```python
from build123d import *

# Parameters (mm, degrees)
F0_W     = 60.96
F0_H     = 31.75
F1_DEPTH = 3.175
F2_R     = 5.08


# Not quite as in the source:
# - a length typed as a fraction of an inch, garbled in the dataset ("3 / 203.2 mm" for 3/8 in), is restored


with BuildPart() as f1:
    # F0 (on Top) → F1 (new body)
    with BuildSketch(Plane.XY):
        Rectangle(F0_W, F0_H)
        with BuildLine():
            Line((-8.128, -4.9660085582), (-8.128, 4.9660085582))
            ThreePointArc((-8.128, 4.9660085582), (0, 9.525), (8.128, 4.9660085582))
            Line((8.128, 4.9660085582), (8.128, -4.9660085582))
            ThreePointArc((8.128, -4.9660085582), (0, -9.525), (-8.128, -4.9660085582))
        make_face(mode=Mode.SUBTRACT)
    extrude(amount=F1_DEPTH)

    # F2
    f2_edges = [f1.edges().sort_by_distance(p)[0] for p in [
        (-30.48, 15.875, 1.5875),
        (30.48, 15.875, 1.5875),
        (-30.48, -15.875, 1.5875),
        (30.48, -15.875, 1.5875),
    ]]
    fillet(f2_edges, radius=F2_R)


solid = f1.part
```
Check sheet for the modelled part. Datum: model origin and axes. Units: mm. A direction names the side the tool comes from. Coordinates: 2 decimals unless noted, no trailing zeros. Order: outer loops, then holes, each group sorted by start corner. A loop starts at its lowest first (then second) coordinate and runs counter-clockwise, first axis right, second up. Notation, with made-up numbers: M -29,5 L 4,5 A25 ccw 4,43 Z; hole C 48,1.25 d8. An arc over 180 degrees is marked long. One line per question, with ' | ' between items. Start each with the question number.
Item 1: Sectioned sample at B-B on y = 6. Record the cut outline in (x, z) (3 decimals).
Item 2: Material ranges on line 1 (X direction, y = 0, z = 0.25); line 2 (Y direction, x = -1, z = 0.8) (3 decimals); line 3 (Y direction, x = 7.5, z = 2.85) (3 decimals), recorded low to high.
Item 3: Sectioned sample at D-D on y = -14. Record the cut outline in (x, z) (3 decimals), and give its area (3 significant figures).
Item 4: Sectioned sample at A-A on z = 1.1. Record the cut outline in (x, y) (3 decimals).
Item 5: Mould release check, pull along X, two halves, no side actions. Record for faces 1 (the cylindrical face through (0.136, -9.524, 1.565)), 2 (the cylindrical face through (-29.03, -14.35, 1.61)), 3 (the cylindrical face through (28.95, 14.43, 1.61)): pulls with the +X half, pulls with the -X half, needs draft (parallel to the pull), parting line crosses it, or undercut.
Item 6: Sectioned sample at C-C on x = 3.5. Record the cut outline in (y, z) (3 decimals), and give its area (3 significant figures).
Item 7: Access from +Z, -Z, +X, -X, +Y, -Y to the whole of each face (thin tool, end or side, straight path). Record for faces 4 (the flat face through (-8.128, 0, 2)), 5 (the flat face through (-7, 7, 3.175)).
Answer below:
1) outline: M -30.48,0 L -7.398,0 L -7.398,3.175 L -30.48,3.175 Z; M 7.398,0 L 30.48,0 L 30.48,3.175 L 7.398,3.175 Z
2) line 1: x = -30.48 to -8.13, 8.13 to 30.48 | line 2: y = -15.875 to -9.472, 9.472 to 15.875 | line 3: y = -15.875 to -5.872, 5.872 to 15.875
3) outline: M -29.341,0 L 29.341,0 L 29.341,3.175 L -29.341,3.175 Z | area: 186 mm^2
4) outline: M -30.48,-10.795 A5.08 ccw -25.4,-15.875 L 25.4,-15.875 A5.08 ccw 30.48,-10.795 L 30.48,10.795 A5.08 ccw 25.4,15.875 L -25.4,15.875 A5.08 ccw -30.48,10.795 Z; hole M -8.128,-4.966 A9.525 ccw 8.128,-4.966 L 8.128,4.966 A9.525 ccw -8.128,4.966 Z
5) face 1: undercut | face 2: pulls with the -X half | face 3: pulls with the +X half
6) outline: M -15.875,0 L -8.859,0 L -8.859,3.175 L -15.875,3.175 Z; M 8.859,0 L 15.875,0 L 15.875,3.175 L 8.859,3.175 Z | area: 44.6 mm^2
7) face 4: +Z, -Z | face 5: +Z, +X, -X, +Y, -Y
